CAD build for the part. Positions are in the model's coordinates, mm. A direction names the side the tool comes from. Give positions to 0.01 mm unless a question says otherwise; leave off trailing zeros. Write each loop counter-clockwise with the first axis right and the second up, starting at its lowest first coordinate (ties: lowest second). Pieces come first, ordered by that corner, then holes. Notation, with made-up numbers: (-14, -16) - (43, -16) arc R22 cw to (43, 23) - close; hole circle Ø8 at (-7, 59). An arc over 180 degrees is marked (long way). Answer as a JSON object with one key per item and string values.
from build123d import *

# Parameters (mm, degrees)
F1_DEPTH = 4.4958
F2_R     = 1.905
F3_DEPTH = 4.4968
F4_W     = 4.4958
F4_H     = 25.4
F4_R     = 9.525
F4_W_2   = 25.4
F4_H_2   = 4.4958
F5_DEPTH = 4.4968


with BuildPart() as f1:
    # F0 (on Top) → F1 (new body)
    with BuildSketch(Plane.XY):
        Polygon((66.04, 76.2), (-66.04, 76.2), (-66.04, 12.7), (-31.75, -76.2), (31.75, -76.2), (66.04, 12.7), align=None)
    extrude(amount=F1_DEPTH)

    # F2 (on face) → F3 (cut, through all)
    with BuildSketch(Plane.XY.offset(4.4958)):
        with Locations((-60.579, 59.3725)):
            Circle(F2_R)
        with Locations((-49.784, 59.3725)):
            Circle(F2_R)
        with Locations((-49.784, 29.5275)):
            Circle(F2_R)
        with Locations((-60.579, 29.5275)):
            Circle(F2_R)
        with Locations((60.579, 59.3725)):
            Circle(F2_R)
        with Locations((49.784, 29.5275)):
            Circle(F2_R)
        with Locations((49.784, 59.3725)):
            Circle(F2_R)
        with Locations((60.579, 29.5275)):
            Circle(F2_R)
    extrude(amount=-F3_DEPTH, mode=Mode.SUBTRACT)

    # F4 (on face) → F5 (cut, through all)
    with BuildSketch(Plane.XY.offset(4.4958)):
        with Locations((-35.9029, 44.45)):
            Rectangle(F4_W, F4_H)
        with Locations((-35.9029, -6.35)):
            Rectangle(F4_W, F4_H)
        with Locations((35.9029, 44.45)):
            Rectangle(F4_W, F4_H)
        with Locations((35.9029, -6.35)):
            Rectangle(F4_W, F4_H)
        with Locations((0, -57.15)):
            Circle(F4_R)
        with Locations((0, -30.7721)):
            Rectangle(F4_W_2, F4_H_2)
    extrude(amount=-F5_DEPTH, mode=Mode.SUBTRACT)


solid = f1.part
(1) Saw through at D-D, the plane z = 1.35. State how many separate pieces and enclosed holes the cut face has, and give its area (3 significant figures).
Answer key:
{"separate pieces": "1", "enclosed holes": "14", "area": "16,100 mm²"}
(2) Saw through at C-C, the plane y = -57.15. Give the cut face in (x, z) (3 decimals), and give its area (3 significant figures).
Answer key:
{"outline": "(-39.098, 0) - (-9.525, 0) - (-9.525, 4.496) - (-39.098, 4.496) - close; (9.525, 0) - (39.098, 0) - (39.098, 4.496) - (9.525, 4.496) - close", "area": "266 mm²"}
(3) Saw through at A-A, the plane y = 36. Give the cut face in (x, z) (3 decimals).
Answer key:
{"outline": "(-66.04, 0) - (-38.151, 0) - (-38.151, 4.496) - (-66.04, 4.496) - close; (-33.655, 0) - (33.655, 0) - (33.655, 4.496) - (-33.655, 4.496) - close; (38.151, 0) - (66.04, 0) - (66.04, 4.496) - (38.151, 4.496) - close"}
(4) Flat gauge pins, fed straight in: P1, Ø2, axis at y = -8.5, z = 1.5, coming from the -X side; P2, Ø1.5, axis at y = -21, z = 1, coming from the -X side; P3, Ø2, axis at y = -7, z = 1, coming from the -X side. Where does each tip first touch, or does it go through?
Answer key:
{"P1": "stops at x = -58.25", "P2": "stops at x = -53.33", "P3": "stops at x = -58.83"}
(5) 3-axis set-ups, long thin cutter, end or side, ignore diameter. For faces 1 (the face through (0, -76.2, 2)), 2 (the face through (36, 57.15, 2)): which of +Z, -Z, +X, -X, +Y, -Y reach the whole face in a straight line?
Answer key:
{"face 1": "+Z, -Z, +X, -X, -Y", "face 2": "+Z, -Z"}
(6) Pull direction Y, two halves, no side cores. Call faces 3 (the face through (33.655, 44, 2)), 4 (the face through (-49.135, -31.128, 2.216)), 5 (the face through (-1, 18, 4.496)), 6 (the face through (1, 76.2, 2)): pulls with the +Y half, pulls with the -Y half, needs draft (parallel to the pull), parting line crosses it, or undercut.
Answer key:
{"face 3": "undercut", "face 4": "pulls with the -Y half", "face 5": "needs draft", "face 6": "pulls with the +Y half"}
(7) Saw through at B-B, the plane x = 0. Give the cut face in (y, z) (3 decimals), and give its area (3 significant figures).
Answer key:
{"outline": "(-76.2, 0) - (-66.675, 0) - (-66.675, 4.496) - (-76.2, 4.496) - close; (-47.625, 0) - (-33.02, 0) - (-33.02, 4.496) - (-47.625, 4.496) - close; (-28.524, 0) - (76.2, 0) - (76.2, 4.496) - (-28.524, 4.496) - close", "area": "579 mm²"}
(8) Probe L1, parallel to X at y = 37, z = 0.9 (3 decimals); L2, parallel to Y at x = 2.5, z = 2.25; L3, parallel to Y at x = 10.5, z = 1. List the from-to ranges inside material, lowest first. Write a range as [from, to].
Answer key:
{"L1": "x = [-66.04, -38.151], [-33.655, 33.655], [38.151, 66.04]", "L2": "y = [-76.2, -66.34], [-47.96, -33.02], [-28.52, 76.2]", "L3": "y = [-76.2, -33.02], [-28.52, 76.2]"}
